The model under review builds one solid part; all positions refer to its coordinate system, in mm. Coordinates: 2 decimals unless noted, no trailing zeros. Loops run counter-clockwise (first coordinate to the right, second up) from the corner with the lowest first, then second, coordinate; pieces in that order, holes last. Notation, with made-up numbers: M -25,33 L -15,33 A20 cw -15,64 Z; hole C 28,0.5 d5. An arc over 180 degrees is marked long. Write item = value, one per line. Start each with the question number.
Q1. We need section A-A on y = -2.25. Give the boundary of the cut face in (x, z), and give its area (3 significant figures).
Q2. Wall thickness on probe 1 along X at (y, z) = (2.5, 0); probe 2 along Z at (x, y) = (-0.65, -1); probe 3 along X at (y, z) = (-0.75, -1): over which ranges is each line inside the solid? List them lowest first.
Q3. Mouldability with a two-part tool opening along X and no side actions: class faces 1 (the face through (0.748, -0.084, -0.976)), 2 (the face through (1.36, 0.09, -2.39)), 3 (the face through (-2.52, 6.16, -1.44)) as released by +X, released by -X, zero draft, split by the parting line, or undercut.
Autodesk Inventor part; units mm, degrees
ref_plane "YZ Plane" through (0, 0, 0) normal (1, 0, 0) x (0, 1, 0)
ref_plane "XZ Plane" through (0, 0, 0) normal (0, 1, 0) x (-1, 0, 0)
ref_plane "XY Plane" through (0, 0, 0) normal (0, 0, 1) x (1, 0, 0)
sketch "スケッチ1" plane through (0, 0, 0) normal (1, 0, 0) x (0, 1, 0)
  line L0 (-6.25, 0) -> (6.25, 0)
  line L1 (0, 0) -> (0, 3.1754) construction
  line L2 (-6.0044, 3.1754) -> (-6.25, 2.75)
  line L3 (-6.25, 2.75) -> (-6.25, 0)
  line L4 (-6.0044, 3.1754) -> (6.0044, 3.1754)
  line L5 (6.0044, 3.1754) -> (6.25, 2.75)
  line L6 (6.25, 2.75) -> (6.25, 0)
  dimension "d1" = 2.75
  dimension "d2" = 3.1754
  dimension "d3" = 30
  dimension "d4" = 12.5
revolve "回転1" add sketch "スケッチ1" angle 360 about axis through (0, -6.25, 0) along (0, 1, 0)
sketch "スケッチ2" plane through (0, 6.25, 0) normal (0, 1, 0) x (1, 0, 0)
  line L0 (0, -3.1754) -> (-2.75, -1.5877)
  line L1 (-2.75, -1.5877) -> (-2.75, 1.5877)
  line L2 (-2.75, 1.5877) -> (0, 3.1754)
  line L3 (0, 3.1754) -> (2.75, 1.5877)
  line L4 (2.75, 1.5877) -> (2.75, -1.5877)
  line L5 (2.75, -1.5877) -> (0, -3.1754)
  circle A0 centre (0, 0) radius 3.1754
  point P0 (0, 0)
  point P1 (0, 0)
  point P2 (0, 0)
  point P3 (0, 0)
  point P4 (0, 3.1754)
  point P5 (0, 3.1754)
  point P6 (2.75, -1.5877)
  point P7 (2.75, -1.5877)
extrude "押し出し1" cut sketch "スケッチ2" against normal through all contours A0 L0 | L5 A0 | A0 L1 | L4 A0 | A0 L2 | L3 A0
hole "穴1" at (0, 6.25, 0) direction (0, -1, 0) diameter 2.459 end through all countersink diameter 3 countersink angle 90
mirror "ミラー1" about plane through (0, 0, 0) normal (0, 1, 0) of "穴1"
equation "\"d2\" = 1.1547 * d1"
properties part number "AS-312.5B" material "アセタール樹脂、黒"
Returned:
q1.outline = M -2.75,-1.59 L 0,-3.18 L 2.75,-1.59 L 2.75,1.59 L 0,3.18 L -2.75,1.59 Z; hole C 0,0 d2.46
q1.area = 21.4 mm^2
q2.probe_1 = -2.75 to -1.23, 1.23 to 2.75
q2.probe_2 = -2.8 to -1.04, 1.04 to 2.8
q2.probe_3 = -2.75 to -0.72, 0.72 to 2.75
q3.face_1 = undercut
q3.face_2 = released by +X
q3.face_3 = released by -X
